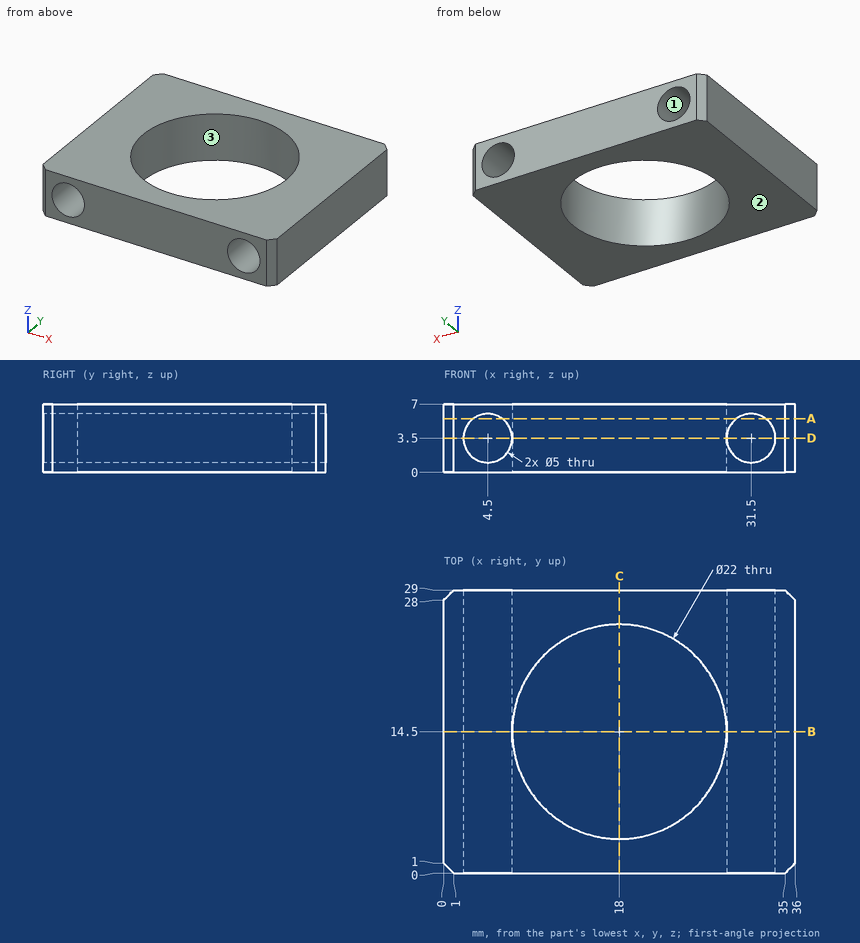
Verification items for this drawing (mm, ordinates from the low corner). Coordinates: 2 decimals unless noted, no trailing zeros. Loops run counter-clockwise (first coordinate to the right, second up) from the corner with the lowest first, then second, coordinate; pieces in that order, holes last. Notation, with made-up numbers: (81.5, 69.5) - (91.5, 69.5) arc R16 ccw to (91.5, 77.5) - close; hole circle Ø5 at (-12.5, 32.25). An arc over 180 degrees is marked (long way). One line per item, written item: value. Start each with the question number.
(1) Cross-section at C-C on x = 18. Enter the section's corners in (y, z).
(2) Cross-section at D-D on z = 3.5. Enter the section's corners in (x, y).
(3) Cross-section at A-A on z = 5.5. Enter the section's corners in (x, y).
(4) Cross-section at B-B on y = 14.5. Enter the section's corners in (x, z), plus the area to 3 significant figures.
(5) Mould release check, pull along Z, two halves, no side actions. Record for the marked faces 1, 2 and 3: released by +Z, released by -Z, zero draft, split by the parting line, or undercut.
(6) Material ranges on line 1 (Z direction, x = 4.5, y = 10.75); line 2 (X direction, y = 20.75, z = 5.75); line 3 (X direction, y = 21.75, z = 5.75), recorded low to high. Write a range as [from, to].
Results below:
1. outline: (0, 0) - (3.5, 0) - (3.5, 7) - (0, 7) - close; (25.5, 0) - (29, 0) - (29, 7) - (25.5, 7) - close
2. outline: (0, 1) - (1, 0) - (2, 0) - (2, 29) - (1, 29) - (0, 28) - close; (7, 0) - (29, 0) - (29, 29) - (7, 29) - close; (34, 0) - (35, 0) - (36, 1) - (36, 28) - (35, 29) - (34, 29) - close; hole circle Ø22 at (18, 14.5)
3. outline: (0, 1) - (1, 0) - (3, 0) - (3, 29) - (1, 29) - (0, 28) - close; (6, 0) - (30, 0) - (30, 29) - (6, 29) - close; (33, 0) - (35, 0) - (36, 1) - (36, 28) - (35, 29) - (33, 29) - close; hole circle Ø22 at (18, 14.5)
4. outline: (0, 0) - (7, 0) - (7, 7) - (0, 7) - close; (29, 0) - (36, 0) - (36, 7) - (29, 7) - close; hole circle Ø5 at (4.5, 3.5); hole circle Ø5 at (31.5, 3.5)
4. area: 58.7 mm2
5. face 1: undercut
5. face 2: released by -Z
5. face 3: zero draft
6. line 1: z = [0, 1], [6, 7]
6. line 2: x = [0, 3.41], [5.59, 8.95], [27.05, 30.41], [32.59, 36]
6. line 3: x = [0, 3.41], [5.59, 9.73], [26.27, 30.41], [32.59, 36]
